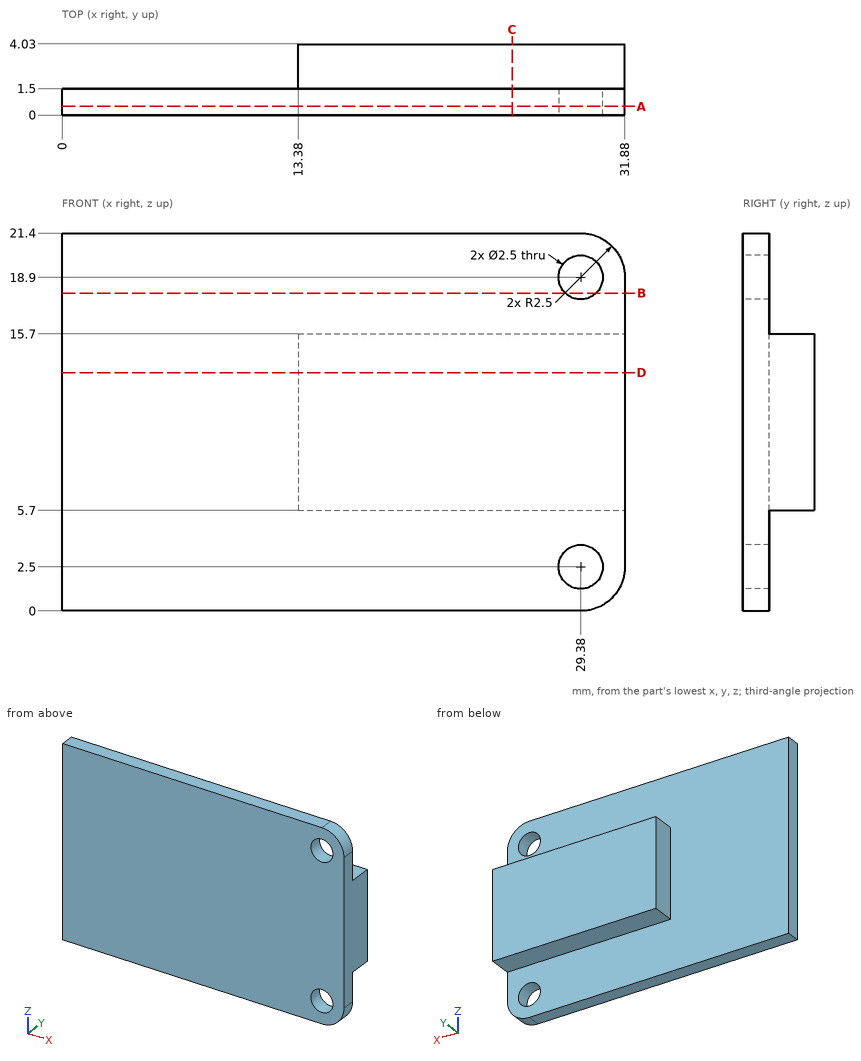
Here's the drawing with two shaded views (mm, measured from the low corner). I have some questions. Give positions to 0.01 mm unless a question says otherwise; leave off trailing zeros. Loops run counter-clockwise (first coordinate to the right, second up) from the corner with the lowest first, then second, coordinate; pieces in that order, holes last. Notation, with made-up numbers: M 73.25,35.25 L 98.25,35.25 A26 cw 98.25,58.25 Z; hole C -36,29.5 d5. An arc over 180 degrees is marked long. Use one line per item in the form item = value. Start each with the question number.
Q1. If we section it at C-C (x = 25.5): Write out the boundary of the cut face in (y, z), then the cut area to 3 significant figures.
Q2. If we section it at B-B (z = 18): Write out the boundary of the cut face in (x, y), then the cut area to 3 significant figures.
Q3. Will these pins go through, and if not, where does the flat tip stop? pin 1 Ø4 at (x, z) = (29.38, 2.5) entering from +Y; pin 2 Ø1.3 at (x, y) = (25, 3) entering from +Z; pin 3 Ø1.5 at (y, z) = (2.5, 18.5) entering from -X; pin 4 Ø1.3 at (x, y) = (23, 3) entering from -Z.
Q4. If we section it at D-D (z = 13.5): Write out the boundary of the cut face in (x, y).
Q5. I need wall thicknesses on line 1 along Z through (x, y) = (29.38, 0.7); line 2 along X through (y, z) = (0.3, 18.9); line 3 along Y through (x, z) = (7, 16.5). Which ranges of each line are inside material? Lowest first, please.
Q6. If we section it at A-A (y = 0.5): Write out the boundary of the cut face in (x, z), then the cut area to 3 significant figures.
Taken from the geometry:
q1.outline = M 0,0 L 1.5,0 L 1.5,5.7 L 4.03,5.7 L 4.03,15.7 L 1.5,15.7 L 1.5,21.4 L 0,21.4 Z
q1.area = 57.4 mm^2
q2.outline = M 0,0 L 28.51,0 L 28.51,1.5 L 0,1.5 Z; M 30.25,0 L 31.88,0 L 31.88,1.5 L 30.25,1.5 Z
q2.area = 45.2 mm^2
q3.pin_1 = 1.5
q3.pin_2 = 15.7
q3.pin_3 = through
q3.pin_4 = 5.7
q4.outline = M 0,0 L 31.88,0 L 31.88,4.03 L 13.38,4.03 L 13.38,1.5 L 0,1.5 Z
q5.line_1 = 0 to 1.25, 3.75 to 17.65, 20.15 to 21.4
q5.line_2 = 0 to 28.13, 30.63 to 31.88
q5.line_3 = 0 to 1.5
q6.outline = M 0,0 L 29.38,0 A2.5 ccw 31.88,2.5 L 31.88,18.9 A2.5 ccw 29.38,21.4 L 0,21.4 Z; hole C 29.38,2.5 d2.5; hole C 29.38,18.9 d2.5
q6.area = 670 mm^2
